from build123d import *

# Parameters (mm, degrees)
SKETCH_1_W      = 2
SKETCH_1_H      = 40
SKETCH_1_W_2    = 40
SKETCH_1_H_2    = 2
SKETCH_1_W_3    = 50
SKETCH_1_R      = 15
SKETCH_1_W_4    = 30
EXTRUDE_3_DEPTH = 2
EXTRUDE_4_DEPTH = 10


with BuildPart() as part:
    # 草图1 → 凸台-拉伸3 (new body)
    with BuildSketch(Plane(origin=(0, 0, 0), x_dir=(0, 0, -1), z_dir=(1, 0, 0))):
        with BuildLine():
            Line((350, 51), (0, 51))
            ThreePointArc((0, 51), (-51, 0), (0, -51))
            Line((0, -51), (350, -51))
            Line((350, -51), (350, -20))
            Line((350, -20), (352, -20))
            Line((352, -20), (352, 20))
            Line((352, 20), (350, 20))
            Line((350, 20), (350, 51))
        make_face()
        with BuildLine():
            ThreePointArc((145, 39), (146.757359313, 43.242640687), (151, 45))
            Line((151, 45), (235, 45))
            Line((235, 45), (235, 45.8))
            Line((235, 45.8), (305, 45.8))
            Line((305, 45.8), (305, 45))
            Line((305, 45), (325.5, 45))
            ThreePointArc((325.5, 45), (329.742640687, 43.242640687), (331.5, 39))
            Line((331.5, 39), (331.5, 31))
            Line((331.5, 31), (151, 31))
            ThreePointArc((151, 31), (146.757359313, 32.757359313), (145, 37))
            Line((145, 37), (145, 39))
        make_face(mode=Mode.SUBTRACT)
        with Locations((1, 0)):
            Rectangle(SKETCH_1_W, SKETCH_1_H, mode=Mode.SUBTRACT)
        with Locations((60, -41)):
            Rectangle(SKETCH_1_W_2, SKETCH_1_H_2, mode=Mode.SUBTRACT)
        with BuildLine():
            Line((97.931678324, -20), (32.068321676, -20))
            ThreePointArc((32.068321676, -20), (30.600998265, -18.811387231), (31.459113977, -17.129282677))
            Line((31.459113977, -17.129282677), (64.390792301, -2.4929812))
            ThreePointArc((64.390792301, -2.4929812), (65, -2.363698523), (65.609207699, -2.4929812))
            Line((65.609207699, -2.4929812), (98.540886023, -17.129282677))
            ThreePointArc((98.540886023, -17.129282677), (99.399001735, -18.811387231), (97.931678324, -20))
        make_face(mode=Mode.SUBTRACT)
        with BuildLine():
            Line((135, -17.39868764), (135, 7.388444501))
            ThreePointArc((135, 7.388444501), (135.75290891, 8.68915773), (137.255806538, 8.684112853))
            Line((137.255806538, 8.684112853), (158.585016393, -3.757926229))
            ThreePointArc((158.585016393, -3.757926229), (159.329207689, -5.056143052), (158.580609404, -6.35182365))
            Line((158.580609404, -6.35182365), (137.25139955, -18.69691671))
            ThreePointArc((137.25139955, -18.69691671), (135.750700102, -18.698129698), (135, -17.39868764))
        make_face(mode=Mode.SUBTRACT)
        with Locations((175, -41)):
            Rectangle(SKETCH_1_W_3, SKETCH_1_H_2, mode=Mode.SUBTRACT)
        with Locations((295, -41)):
            Rectangle(SKETCH_1_W_3, SKETCH_1_H_2, mode=Mode.SUBTRACT)
        with BuildLine():
            Line((189.451619145, -25), (145.548380855, -25))
            ThreePointArc((145.548380855, -25), (144.100364535, -23.891469969), (144.792574317, -22.204331649))
            Line((144.792574317, -22.204331649), (166.744193462, -9.399220481))
            ThreePointArc((166.744193462, -9.399220481), (167.5, -9.194888832), (168.255806538, -9.399220481))
            Line((168.255806538, -9.399220481), (190.207425683, -22.204331649))
            ThreePointArc((190.207425683, -22.204331649), (190.899635465, -23.891469969), (189.451619145, -25))
        make_face(mode=Mode.SUBTRACT)
        with BuildLine():
            ThreePointArc((197.744193462, 8.684112853), (199.24709109, 8.68915773), (200, 7.388444501))
            Line((200, 7.388444501), (200, -17.388444501))
            ThreePointArc((200, -17.388444501), (199.24709109, -18.68915773), (197.744193462, -18.684112853))
            Line((197.744193462, -18.684112853), (176.506860031, -6.295668351))
            ThreePointArc((176.506860031, -6.295668351), (175.762666569, -5), (176.506860031, -3.704331649))
            Line((176.506860031, -3.704331649), (197.744193462, 8.684112853))
        make_face(mode=Mode.SUBTRACT)
        with Locations((232.5, -5)):
            Circle(SKETCH_1_R, mode=Mode.SUBTRACT)
        with BuildLine():
            Line((319.974166797, -25.394327939), (276.070928507, -25.394327939))
            ThreePointArc((276.070928507, -25.394327939), (274.622912187, -24.285797907), (275.315121969, -22.598659587))
            Line((275.315121969, -22.598659587), (297.266741114, -9.793548419))
            ThreePointArc((297.266741114, -9.793548419), (298.022547652, -9.589216771), (298.778354191, -9.793548419))
            Line((298.778354191, -9.793548419), (320.729973336, -22.598659587))
            ThreePointArc((320.729973336, -22.598659587), (321.422183118, -24.285797907), (319.974166797, -25.394327939))
        make_face(mode=Mode.SUBTRACT)
        with BuildLine():
            Line((265.522547652, -17.793015579), (265.522547652, 6.994116563))
            ThreePointArc((265.522547652, 6.994116563), (266.275456563, 8.294829792), (267.778354191, 8.289784914))
            Line((267.778354191, 8.289784914), (289.107564045, -4.152254168))
            ThreePointArc((289.107564045, -4.152254168), (289.851755342, -5.45047099), (289.103157056, -6.746151588))
            Line((289.103157056, -6.746151588), (267.773947202, -19.091244648))
            ThreePointArc((267.773947202, -19.091244648), (266.273247754, -19.092457637), (265.522547652, -17.793015579))
        make_face(mode=Mode.SUBTRACT)
        with BuildLine():
            ThreePointArc((327.730104505, 8.28146303), (329.239985391, 8.298885363), (330, 6.994116563))
            Line((330, 6.994116563), (330, -17.477952976))
            ThreePointArc((330, -17.477952976), (329.24709109, -18.778666205), (327.744193462, -18.773621327))
            Line((327.744193462, -18.773621327), (307.029407683, -6.68999629))
            ThreePointArc((307.029407683, -6.68999629), (306.285236534, -5.40250951), (307.015318726, -4.106981472))
            Line((307.015318726, -4.106981472), (327.730104505, 8.28146303))
        make_face(mode=Mode.SUBTRACT)
        with BuildLine():
            Line((15, -7.691857033), (15, 17.691857033))
            ThreePointArc((15, 17.691857033), (15.682629689, 18.94959539), (17.109207699, 19.062574356))
            Line((17.109207699, 19.062574356), (45.665886023, 6.370717323))
            ThreePointArc((45.665886023, 6.370717323), (46.556678324, 5), (45.665886023, 3.629282677))
            Line((45.665886023, 3.629282677), (17.109207699, -9.062574356))
            ThreePointArc((17.109207699, -9.062574356), (15.682629689, -8.94959539), (15, -7.691857033))
        make_face(mode=Mode.SUBTRACT)
        with BuildLine():
            Line((112.890792301, -9.062574356), (84.334113977, 3.629282677))
            ThreePointArc((84.334113977, 3.629282677), (83.443321676, 5), (84.334113977, 6.370717323))
            Line((84.334113977, 6.370717323), (112.890792301, 19.062574356))
            ThreePointArc((112.890792301, 19.062574356), (114.317370311, 18.94959539), (115, 17.691857033))
            Line((115, 17.691857033), (115, -7.691857033))
            ThreePointArc((115, -7.691857033), (114.317370311, -8.94959539), (112.890792301, -9.062574356))
        make_face(mode=Mode.SUBTRACT)
        with BuildLine():
            ThreePointArc((31.459113977, 27.129282677), (30.600998265, 28.811387231), (32.068321676, 30))
            Line((32.068321676, 30), (97.931678324, 30))
            ThreePointArc((97.931678324, 30), (99.399001735, 28.811387231), (98.540886023, 27.129282677))
            Line((98.540886023, 27.129282677), (65.609207699, 12.4929812))
            ThreePointArc((65.609207699, 12.4929812), (65, 12.363698523), (64.390792301, 12.4929812))
            Line((64.390792301, 12.4929812), (31.459113977, 27.129282677))
        make_face(mode=Mode.SUBTRACT)
        with BuildLine():
            ThreePointArc((144.792574317, 12.204331649), (144.100364535, 13.891469969), (145.548380855, 15))
            Line((145.548380855, 15), (189.885145799, 15))
            ThreePointArc((189.885145799, 15), (191.333825129, 13.889009252), (190.636545348, 12.20177093))
            Line((190.636545348, 12.20177093), (168.381459159, -0.679208343))
            ThreePointArc((168.381459159, -0.679208343), (167.627511138, -0.880977109), (166.874253072, -0.676647625))
            Line((166.874253072, -0.676647625), (144.792574317, 12.204331649))
        make_face(mode=Mode.SUBTRACT)
        with BuildLine():
            ThreePointArc((275.298059327, 12.21443661), (274.625531488, 13.901032988), (276.070928507, 15))
            Line((276.070928507, 15), (321.088992758, 15))
            ThreePointArc((321.088992758, 15), (322.537672089, 13.889009252), (321.840392308, 12.20177093))
            Line((321.840392308, 12.20177093), (298.904006812, -1.073536282))
            ThreePointArc((298.904006812, -1.073536282), (298.140143671, -1.275255431), (297.379738082, -1.060870603))
            Line((297.379738082, -1.060870603), (275.298059327, 12.21443661))
        make_face(mode=Mode.SUBTRACT)
        Polygon((-40, 20), (-9.698170842, 42.091834457), (-8.519939671, 40.475736902), (-38.821768829, 18.383902445), align=None, mode=Mode.SUBTRACT)
        with Locations((-25, -9)):
            Rectangle(SKETCH_1_W_4, SKETCH_1_H_2, mode=Mode.SUBTRACT)
        Polygon((-40, -20), (-38.821768829, -18.383902445), (-8.519939671, -40.475736902), (-9.698170842, -42.091834457), align=None, mode=Mode.SUBTRACT)
    extrude(amount=EXTRUDE_3_DEPTH)

    # 草图2 → 凸台-拉伸4 (add)
    with BuildSketch(Plane(origin=(0, 0, 0), x_dir=(0, 0, -1), z_dir=(1, 0, 0))):
        Polygon((151, 51), (151, 45), (235, 45), (235, 45.8), (305, 45.8), (305, 45), (325.5, 45), (325.5, 51), align=None)
        Polygon((325.5, 31), (151, 31), (151, 24), (325.5, 23.560383637), align=None)
    extrude(amount=-EXTRUDE_4_DEPTH)


solid = part.part
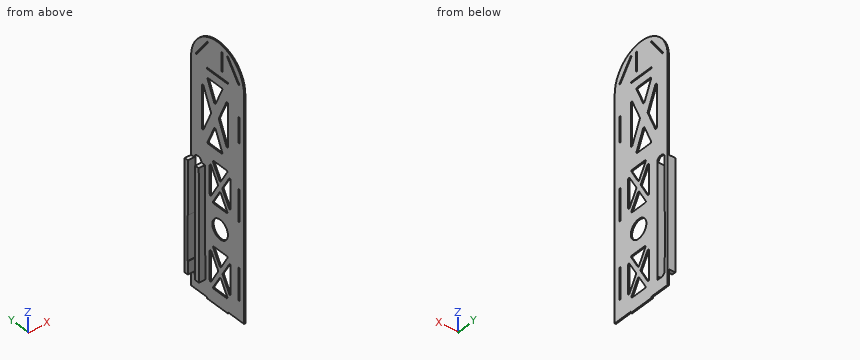
Input: part model. Units: mm. Frame: model coordinates. Round coordinates to 2 decimals unless told otherwise and drop trailing zeros. Write each loop counter-clockwise with the first axis right and the second up, starting at its lowest first coordinate (ties: lowest second). Pieces come first, ordered by that corner, then holes.
1) Cut plane C-C (z = 24.5). Return the cut outline in (x, y).
2) Ray query, L1, parallel to Y at x = 0.7, z = -232.5; L2, parallel to X at y = -10, z = -103; L3, parallel to Y at x = -2.5, z = -175. Return the intervals inside material, ascending.
3) Cut plane B-B (z = -254). Return the cut outline in (x, y).
4) Contact query for flat-ended pins moving along their axis: P1, Ø0.9, axis at x = -6.5, y = 45.5, coming from the +Z side; P2, Ø1, axis at x = 0.5, y = 34.5, coming from the +Z side; P3, Ø3, axis at y = 34, z = -95, coming from the -X side; P4, Ø4, axis at x = -2.5, z = -118, coming from the +Y side. Output: stop coordinate, or through.
5) Cut plane A-A (x = -6.75). Return the cut outline in (y, z), then the cut area to 3 significant figures.
Geometry says:
1. outline: (0, -44.73) - (2, -44.73) - (2, -31.3) - (0, -31.3) - close; (0, -28.83) - (2, -28.83) - (2, -10) - (0, -10) - close; (0, -8) - (2, -8) - (2, 28.83) - (0, 28.83) - close; (0, 31.3) - (2, 31.3) - (2, 44.73) - (0, 44.73) - close
2. L1: y = -51 to -20, 10 to 31, 45 to 51
2. L2: x = 0 to 2
2. L3: y = 23.94 to 31, 45 to 51
3. outline: (-10, 23.74) - (0, 23.74) - (0, -51) - (2, -51) - (2, 31) - (-10, 31) - close; (-10, 45.8) - (2, 45.8) - (2, 51) - (-10, 51) - close
4. P1: stops at z = -151
4. P2: stops at z = 38.01
4. P3: stops at x = 0
4. P4: passes through
5. outline: (23.56, -325.5) - (31, -325.5) - (31, -151) - (24, -151) - close; (45, -325.5) - (51, -325.5) - (51, -151) - (45, -151) - (45, -235) - (45.8, -235) - (45.8, -305) - (45, -305) - close
5. area: 2,250 mm2
